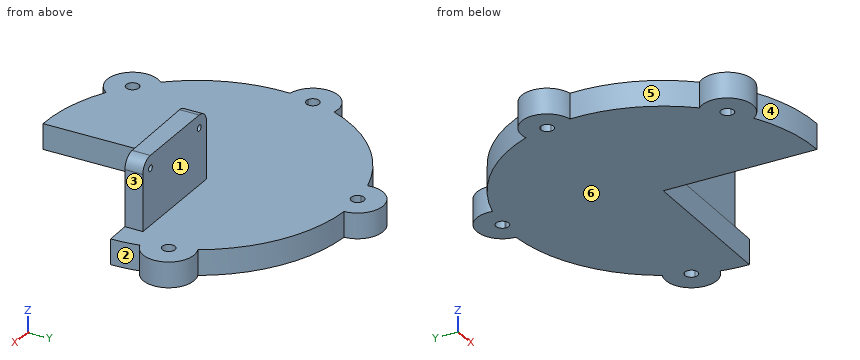
from build123d import *

# Parameters (mm, degrees)
F1_DEPTH = 3.175
F3_DEPTH = 8.636
F4_R     = 1.6002
F5_R     = 0.3937
F6_DEPTH = 25.4
F7_DEPTH = 25.4


with BuildPart() as f1:
    # F0 (on Top) → F1 (new body)
    with BuildSketch(Plane.XY):
        with BuildLine():
            ThreePointArc((31.2392285465, -28.7320576953), (35.8370397612, -30.5372732521), (40.7444173623, -31.0996932487))
            Line((40.7444173623, -31.0996932487), (40.4414878789, -12.0521019645))
            Line((40.4414878789, -12.0521019645), (59.489079163, -11.7491724811))
            ThreePointArc((59.489079163, -11.7491724811), (59.3824551279, -10.0168477616), (59.1186092237, -8.3014169243))
            ThreePointArc((59.1186092237, -8.3014169243), (58.8457012348, -7.1340301115), (58.4999035926, -5.9861212597))
            ThreePointArc((58.4999035926, -5.9861212597), (57.3481289048, -5.5817963761), (57.9356764569, -4.5118190787))
            ThreePointArc((57.9356764569, -4.5118190787), (57.4267405613, -3.4263445302), (56.8505347882, -2.3750321845))
            ThreePointArc((56.8505347882, -2.3750321845), (50.3338026609, 4.2280887055), (41.4709261237, 6.9700629202))
            ThreePointArc((41.4709261237, 6.9700629202), (40.2797629673, 6.9972115416), (39.0892324485, 6.949842811))
            ThreePointArc((39.0892324485, 6.949842811), (39.096904661, 6.8862640952), (39.0994675382, 6.822275443))
            ThreePointArc((39.0994675382, 6.822275443), (38.3257250063, 6.0226097042), (37.5010041114, 6.7695891182))
            ThreePointArc((37.5010041114, 6.7695891182), (36.33013815, 6.5489545487), (35.1753550199, 6.2555561247))
            ThreePointArc((35.1753550199, 6.2555561247), (27.5701803077, 1.991827023), (22.66118966, -5.2137179999))
            ThreePointArc((22.66118966, -5.2137179999), (22.2660417046, -6.3463455408), (21.9429633319, -7.5015976424))
            ThreePointArc((21.9429633319, -7.5015976424), (22.4949706136, -7.7432037883), (22.7218707315, -8.3014169243))
            ThreePointArc((22.7218707315, -8.3014169243), (22.3727631285, -8.9622995673), (21.6300925341, -9.0464564127))
            ThreePointArc((21.6300925341, -9.0464564127), (21.4782165965, -10.2363810963), (21.4015341389, -11.4335055067))
            ThreePointArc((21.4015341389, -11.4335055067), (22.5472730496, -18.5865931952), (26.2806968621, -24.7947271956))
            ThreePointArc((26.2806968621, -24.7947271956), (27.1038904808, -25.6539766753), (27.9791241647, -26.4601549439))
            ThreePointArc((27.9791241647, -26.4601549439), (28.8701686575, -26.1957695514), (29.4100136292, -26.9523588259))
            ThreePointArc((29.4100136292, -26.9523588259), (29.3642656384, -27.2190291398), (29.2322532085, -27.4552041879))
            ThreePointArc((29.2322532085, -27.4552041879), (30.2157917864, -28.1249871885), (31.2392285465, -28.7320576953))
        make_face()
        with BuildLine():
            ThreePointArc((26.2806968621, -24.7947271956), (26.6355383886, -29.438815624), (31.2392285465, -28.7320576953))
            ThreePointArc((31.2392285465, -28.7320576953), (30.2157917864, -28.1249871885), (29.2322532085, -27.4552041879))
            ThreePointArc((29.2322532085, -27.4552041879), (28.1123710686, -27.578945939), (27.9791241647, -26.4601549439))
            ThreePointArc((27.9791241647, -26.4601549439), (27.1038904808, -25.6539766753), (26.2806968621, -24.7947271956))
        make_face()
        with BuildLine():
            ThreePointArc((58.4999035926, -5.9861212597), (58.8457012348, -7.1340301115), (59.1186092237, -8.3014169243))
            ThreePointArc((59.1186092237, -8.3014169243), (61.0606385443, -4.1609894973), (56.8505347882, -2.3750321845))
            ThreePointArc((56.8505347882, -2.3750321845), (57.4267405613, -3.4263445302), (57.9356764569, -4.5118190787))
            ThreePointArc((57.9356764569, -4.5118190787), (58.6015298758, -4.6761681541), (58.895475254, -5.2958192727))
            ThreePointArc((58.895475254, -5.2958192727), (58.7895737608, -5.6936238015), (58.4999035926, -5.9861212597))
        make_face()
        with BuildLine():
            ThreePointArc((22.66118966, -5.2137179999), (18.809946607, -7.6711982175), (21.4015341389, -11.4335055067))
            ThreePointArc((21.4015341389, -11.4335055067), (21.4782165965, -10.2363810963), (21.6300925341, -9.0464564127))
            ThreePointArc((21.6300925341, -9.0464564127), (21.1375910521, -8.1426018102), (21.9429633319, -7.5015976424))
            ThreePointArc((21.9429633319, -7.5015976424), (22.2660417046, -6.3463455408), (22.66118966, -5.2137179999))
        make_face()
        with BuildLine():
            ThreePointArc((39.0892324485, 6.949842811), (40.2797629673, 6.9972115416), (41.4709261237, 6.9700629202))
            ThreePointArc((41.4709261237, 6.9700629202), (37.9413240389, 9.9770226362), (35.1753550199, 6.2555561247))
            ThreePointArc((35.1753550199, 6.2555561247), (36.33013815, 6.5489545487), (37.5010041114, 6.7695891182))
            ThreePointArc((37.5010041114, 6.7695891182), (38.2091405764, 7.6172717357), (39.0892324485, 6.949842811))
        make_face()
    extrude(amount=F1_DEPTH)

    # F2 (on face) → F3 (join)
    with BuildSketch(Plane.XY.offset(3.175)):
        Polygon((42.631557275, -12.0172714927), (56.3164878789, -11.7996288052), (56.3164878789, -9.556004395), (42.5924137235, -9.556004395), align=None)
    extrude(amount=F3_DEPTH)

    # F4
    f4_edges = [f1.edges().sort_by_distance(p)[0] for p in [
        (42.611985, -10.786638, 11.811),
        (56.316488, -10.677817, 11.811),
    ]]
    fillet(f4_edges, radius=F4_R)

    # F5 (on face) → F6 (cut)
    with BuildSketch(Plane(origin=(0.2018523454, -12.6920659276, 0), x_dir=(0.9998735582, 0.0159018102, 0), z_dir=(0.0159018102, -0.9998735582, 0))):
        with Locations((44.0352704953, 10.2108)):
            Circle(F5_R)
    extrude(amount=-F6_DEPTH, mode=Mode.SUBTRACT)

    # F5 (on face) → F7 (cut)
    with BuildSketch(Plane(origin=(0.2018523454, -12.6920659276, 0), x_dir=(0.9998735582, 0.0159018102, 0), z_dir=(0.0159018102, -0.9998735582, 0))):
        with Locations((44.0352704953, 10.2108)):
            Circle(F5_R)
        with Locations((54.5213293072, 10.2108)):
            Circle(F5_R)
    extrude(amount=-F7_DEPTH, mode=Mode.SUBTRACT)


solid = f1.part
CAD build for the part. Positions are in the model's coordinates, mm. Face numbers are marked on the shaded views. A direction names the side the tool comes from. Round coordinates to 2 decimals unless told otherwise and drop trailing zeros. Write each loop counter-clockwise with the first axis right and the second up, starting at its lowest first coordinate (ties: lowest second). Pieces come first, ordered by that corner, then holes.
(1) Slice it at B-B, the plane y = -3.5. Write the cut outline in (x, z) (3 decimals), and give its area (3 significant figures).
(2) Slice it at A-A, the plane z = 0.5. Count the separate pieces of the cut face and the enclosed holes in it, and give its area (3 significant figures).
(3) 3-axis set-ups, long thin cutter, end or side, ignore diameter. For the marked faces 1, 2 and 3: which of +Z, -Z, +X, -X, +Y, -Y reach the whole face in a straight line?
(4) Probe line 1 along Z through (x, y) = (27, -24) (3 decimals); line 2 along Y through (x, z) = (45, 3.5); line 3 along X through (y, z) = (-11.5, 2.75). List the from-to ranges inside material, lowest first.
(5) Slice it at C-C, the plane z = 8.5. Write the cut outline in (x, y).
(6) Mould opens along X. For the marked faces 4, 5 and 6 say: pulls with the +X half, pulls with the -X half, needs draft (parallel to the pull), parting line crosses it, or undercut.
(7) Drop flat-ended pins along their axis: P1, Ø6, axis at x = 45.5, z = 6, coming from the +Y side; P2, Ø6, axis at x = 41, z = 5.5, coming from the +Y side; P3, Ø4, axis at y = -16, z = 3, coming from the -X side. Give the stop position or say it passes through.
From the geometry:
1. outline: (23.419, 0) - (60.714, 0) - (60.714, 3.175) - (23.419, 3.175) - close
1. area: 118 mm2
2. separate pieces: 1
2. enclosed holes: 4
2. area: 910 mm2
3. face 1: +Z, +X, -X, +Y
3. face 2: +Z, -Z, +X
3. face 3: +Z, +X, +Y, -Y
4. line 1: z = 0 to 3.175
4. line 2: y = -11.98 to -9.56
4. line 3: x = 21.4 to 59.48
5. outline: (42.59, -9.56) - (42.63, -12.02) - (56.32, -11.8) - (56.32, -9.56) - close
6. face 4: undercut
6. face 5: pulls with the -X half
6. face 6: needs draft
7. P1: stops at y = 6.56
7. P2: stops at y = 9.89
7. P3: stops at x = 21.49
